The model under review builds one solid part; all positions refer to its coordinate system, in mm. Face numbers are marked on the shaded views. A direction names the side the tool comes from. Round coordinates to 2 decimals unless told otherwise and drop trailing zeros. Write each loop counter-clockwise with the first axis right and the second up, starting at its lowest first coordinate (ties: lowest second). Pieces come first, ordered by that corner, then holes. Notation, with made-up numbers: M -23,-27 L 30,-27 A23 ccw 30,-3 Z; hole C 77,47.5 d2. An arc over 180 degrees is marked long. Write item = value, one per line. Start each with the question number.
Item 1: To check wall thickness, follow line 1 along Y through (x, z) = (0, 6.2); line 2 along Y through (x, z) = (0, 5.75); line 3 along Y through (x, z) = (0, 3). State the ranges of each line that lie inside material, in increasing order.
Item 2: The part is to be moulded in two halves that separate along X. For the marked faces 3, 4, 5 and 6, say which applies: +X half, -X half, draft (parallel to the pull), parting line (faces both ways), or undercut.
Item 3: Take a section at D-D, the plane y = 4. Give the boundary of the cut face in (x, z), plus the area to 3 significant figures.
Item 4: Take a section at B-B, the plane z = 3.5. Give the boundary of the cut face in (x, y).
Item 5: Take a section at A-A, the plane x = 0. Give the boundary of the cut face in (y, z).
Item 6: For pin 1 Ø2 at (x, z) = (6.5, 6) entering from -Y; pin 2 Ø9.5 at (x, y) = (0, 0) entering from -Z; pin 3 Ø4 at (x, z) = (-6.5, 5.5) entering from +Y, all flat-tipped, find the tip position at first contact; note any pin that passes through.
Item 7: Take a section at C-C, the plane y = 0.5. Give the boundary of the cut face in (x, z).
Item 8: Tool access review of the marked faces 1 and 2: name each direction out of +Z, -Z, +X, -X, +Y, -Y from which nothing blocks a thin tool from reaching the whole face with its end or side.
from build123d import *

# Parameters (mm, degrees)
CYLINDER001_R           = 4
CYLINDER001_DEPTH       = 70
CYLINDER001_PITCH_ANGLE = 90
CYLINDER_R              = 15
CYLINDER_DEPTH          = 8
SKETCH_R                = 3
POCKET_DEPTH            = 8.001
POCKET001_DEPTH         = 4


with BuildPart() as cylinder001:
    # Cylinder001 → Cylinder001 (new body)
    with BuildSketch(Plane.XY):
        Circle(CYLINDER001_R)
    extrude(amount=CYLINDER001_DEPTH)


with BuildPart() as cylinder001_1:
    # Cylinder001 pitch: moved
    add(cylinder001.part.rotate(Axis((0, 0, 0), (0, 1, 0)), CYLINDER001_PITCH_ANGLE))


with BuildPart() as cylinder001_2:
    # Cylinder001 placement: moved
    add(cylinder001_1.part.moved(Location((-35.24, -8.5813, 8.7367))))


with BuildPart() as pocket001:
    # Cylinder → Cylinder (new body)
    with BuildSketch(Plane.XY):
        Circle(CYLINDER_R)
    extrude(amount=CYLINDER_DEPTH)

    # Sketch → Pocket (cut, through all)
    with BuildSketch(Plane.XY.offset(8)):
        Circle(SKETCH_R)
    extrude(amount=-POCKET_DEPTH, mode=Mode.SUBTRACT)

    # Cut: cut Cylinder001
    add(cylinder001_2.part, mode=Mode.SUBTRACT)

    # Sketch001 → Pocket001 (cut)
    with BuildSketch(Plane(origin=(0, 0, 0), x_dir=(1, 0, 0), z_dir=(0, 0, -1))):
        Polygon((3.464102, -6), (6.928203, 0), (3.464102, 6), (-3.464102, 6), (-6.928203, 0), (-3.464102, -6), align=None)
    extrude(amount=-POCKET001_DEPTH, mode=Mode.SUBTRACT)


solid = pocket001.part
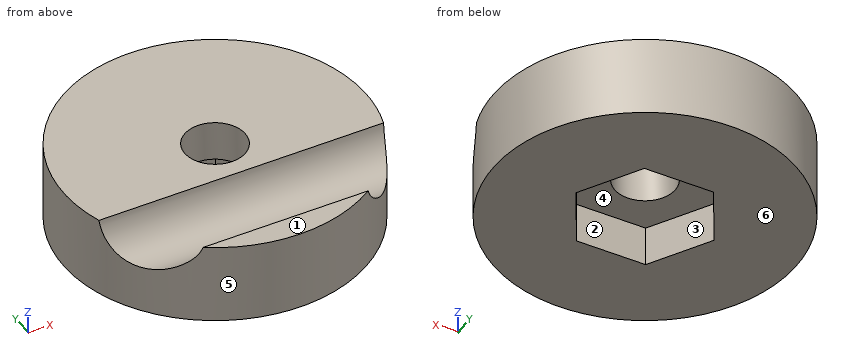
Response values:
q1.line_1 = -15 to -11.67, -5.49 to -3, 3 to 15
q1.line_2 = -15 to -11.24, -5.92 to -3, 3 to 15
q1.line_3 = -15 to -6, 6 to 15
q2.face_3 = undercut
q2.face_4 = undercut
q2.face_5 = parting line
q2.face_6 = draft
q3.outline = M -14.46,0 L -4.62,0 L -4.62,4 L 4.62,4 L 4.62,0 L 14.46,0 L 14.46,8 L -14.46,8 Z
q3.area = 194 mm2
q4.outline = C 0,0 d30; hole M -6.93,0 L -3.46,-6 L 3.46,-6 L 6.93,0 L 3.46,6 L -3.46,6 Z
q5.outline = M -15,0 L -6,0 L -6,4 L -3,4 L -3,8 L -4.65,8 A4 cw -12.51,8 L -15,8 Z; M 3,4 L 6,4 L 6,0 L 15,0 L 15,8 L 3,8 Z
q6.pin_1 = -13.96
q6.pin_2 = 4
q6.pin_3 = 14.31
q7.outline = M -14.99,0 L -6.64,0 L -6.64,4 L -2.96,4 L -2.96,8 L -14.99,8 Z; M 2.96,4 L 6.64,4 L 6.64,0 L 14.99,0 L 14.99,8 L 2.96,8 Z
q8.face_1 = +Z, +X, -X, +Y, -Y
q8.face_2 = -Z
